from build123d import *

# Parameters (mm, degrees)
SKETCH1_W                    = 60
SKETCH1_H                    = 170
BASE_FLANGE1_DEPTH           = 4
EDGE_FLANGE1_STRIP_W         = 26
EDGE_FLANGE1_STRIP_H         = 4
EDGE_FLANGE1_STRIP_CUT_DEPTH = 170
EDGE_FLANGE1_DEPTH           = 170
SKETCH15_R                   = 15
SKETCH15_R_2                 = 10
CUT_EXTRUDE4_DEPTH           = 10
CUT_EXTRUDE5_DEPTH           = 10
SKETCH31_R                   = 2.6
CUT_EXTRUDE9_DEPTH           = 7
FILLET1_R                    = 10
SKETCH32_R                   = 1.6
CUT_EXTRUDE10_DEPTH          = 10
F_1_0MM_DOWEL_HOLE2_D        = 5.2
F_1_0MM_DOWEL_HOLE2_DEPTH    = 12.03
F_1_0MM_DOWEL_HOLE2_TIP      = 1.562237609
F_1_0MM_DOWEL_HOLE3_D        = 5.2
F_1_0MM_DOWEL_HOLE3_DEPTH    = 12.03
F_1_0MM_DOWEL_HOLE3_TIP      = 1.562237609
CUT_EXTRUDE11_DEPTH          = 10


# Sheet-metal steps are written as plain solids
with BuildPart() as part:
    # Sketch1 → Base-Flange1 (new body)
    with BuildSketch(Plane(origin=(0, 0, 0), x_dir=(1, 0, 0), z_dir=(0, 1, 0))):
        Rectangle(SKETCH1_W, SKETCH1_H)
    extrude(amount=-BASE_FLANGE1_DEPTH)

    # Edge-Flange1 strip (across the edge) → Edge-Flange1 strip cut (cut)
    with BuildSketch(Plane(origin=(30, 0, 85), x_dir=(-1, 0, 0), z_dir=(0, 0, -1))):
        with Locations((-8, -2)):
            Rectangle(EDGE_FLANGE1_STRIP_W, EDGE_FLANGE1_STRIP_H)
    extrude(amount=EDGE_FLANGE1_STRIP_CUT_DEPTH, mode=Mode.SUBTRACT)

    # Edge-Flange1 section (across the edge) → Edge-Flange1 (add)
    with BuildSketch(Plane(origin=(30, 0, 85), x_dir=(-1, 0, 0), z_dir=(0, 0, -1))):
        with BuildLine():
            Line((-4, 5), (-4, 186))
            Line((-4, 186), (0, 186))
            Line((0, 186), (0, 5))
            ThreePointArc((0, 5), (1.464466094, 1.464466094), (5, 0))
            Line((5, 0), (5, -4))
            ThreePointArc((5, -4), (-1.363961031, -1.363961031), (-4, 5))
        make_face()
    extrude(amount=EDGE_FLANGE1_DEPTH)

    # Sketch15 → Cut-Extrude4 (cut)
    with BuildSketch(Plane(origin=(34, 0, 0), x_dir=(0, 0, -1), z_dir=(1, 0, 0))):
        with Locations(Location((-43, 63, 0), (0, 0, 90))):
            Circle(SKETCH15_R)
        with Locations(Location((57, 143, 0), (0, 0, 90))):
            Circle(SKETCH15_R_2)
    extrude(amount=-CUT_EXTRUDE4_DEPTH, mode=Mode.SUBTRACT)

    # Sketch16 → Cut-Extrude5 (cut)
    with BuildSketch(Plane(origin=(34, 0, 0), x_dir=(0, 0, -1), z_dir=(1, 0, 0))):
        Polygon((-85, 186), (-85, 96), (45, 186), align=None)
    extrude(amount=-CUT_EXTRUDE5_DEPTH, mode=Mode.SUBTRACT)

    # Sketch31 → Cut-Extrude9 (cut)
    with BuildSketch(Plane.ZY.offset(-30)):
        with Locations(Location((76, 61.5, 0), (0, 0, 270))):
            Circle(SKETCH31_R)
        with Locations(Location((10, 61.5, 0), (0, 0, 270))):
            Circle(SKETCH31_R)
        with Locations(Location((43, 23, 0), (0, 0, 270))):
            Circle(SKETCH31_R)
    extrude(amount=-CUT_EXTRUDE9_DEPTH, mode=Mode.SUBTRACT)

    # Fillet1
    fillet1_edges = [part.edges().sort_by_distance(p)[0] for p in [
        (32, 186, -85),
        (32, 186, -45),
        (32, 96, 85),
        (-30, -2, 85),
        (-30, -2, -85),
    ]]
    fillet(fillet1_edges, radius=FILLET1_R)

    # Sketch32 → Cut-Extrude10 (cut)
    with BuildSketch(Plane.ZY.offset(-30)):
        with Locations(Location((-74.67766953, 143, 0), (0, 0, 270))):
            Circle(SKETCH32_R)
        with Locations(Location((-57, 125.32233047, 0), (0, 0, 270))):
            Circle(SKETCH32_R)
        with Locations(Location((-39.32233047, 143, 0), (0, 0, 270))):
            Circle(SKETCH32_R)
        with Locations(Location((-57, 160.67766953, 0), (0, 0, 270))):
            Circle(SKETCH32_R)
    extrude(amount=-CUT_EXTRUDE10_DEPTH, mode=Mode.SUBTRACT)

    # Ø1.0mm Dowel Hole2
    with Locations(Plane(origin=(34, 0, 0), x_dir=(0, 0, -1), z_dir=(1, 0, 0))):
        with Locations((-72.5, 26), (72.5, 26), (72.5, 116), (-22.5, 101), (59.5, 178)):
            Hole(F_1_0MM_DOWEL_HOLE2_D / 2, depth=F_1_0MM_DOWEL_HOLE2_DEPTH)
            with Locations((0, 0, -(F_1_0MM_DOWEL_HOLE2_DEPTH + F_1_0MM_DOWEL_HOLE2_TIP / 2))):  # 118° drill point
                Cone(0, F_1_0MM_DOWEL_HOLE2_D / 2, F_1_0MM_DOWEL_HOLE2_TIP, mode=Mode.SUBTRACT)

    # Ø1.0mm Dowel Hole3
    with Locations(Plane(origin=(0, 0, 0), x_dir=(1, 0, 0), z_dir=(0, 1, 0))):
        with Locations((-15, 70), (-15, 0), (-15, -70)):
            Hole(F_1_0MM_DOWEL_HOLE3_D / 2, depth=F_1_0MM_DOWEL_HOLE3_DEPTH)
            with Locations((0, 0, -(F_1_0MM_DOWEL_HOLE3_DEPTH + F_1_0MM_DOWEL_HOLE3_TIP / 2))):  # 118° drill point
                Cone(0, F_1_0MM_DOWEL_HOLE3_D / 2, F_1_0MM_DOWEL_HOLE3_TIP, mode=Mode.SUBTRACT)

    # Sketch40 → Cut-Extrude11 (cut)
    with BuildSketch(Plane(origin=(0, 0, 0), x_dir=(1, 0, 0), z_dir=(0, 1, 0))):
        with BuildLine():
            Line((-19, -72.6), (-11, -72.6))
            ThreePointArc((-11, -72.6), (-8.4, -70), (-11, -67.4))
            Line((-11, -67.4), (-19, -67.4))
            ThreePointArc((-19, -67.4), (-21.6, -70), (-19, -72.6))
        make_face()
        with BuildLine():
            Line((-19, -2.6), (-11, -2.6))
            ThreePointArc((-11, -2.6), (-8.4, 0), (-11, 2.6))
            Line((-11, 2.6), (-19, 2.6))
            ThreePointArc((-19, 2.6), (-21.6, 0), (-19, -2.6))
        make_face()
        with BuildLine():
            Line((-19, 67.4), (-11, 67.4))
            ThreePointArc((-11, 67.4), (-8.4, 70), (-11, 72.6))
            Line((-11, 72.6), (-19, 72.6))
            ThreePointArc((-19, 72.6), (-21.6, 70), (-19, 67.4))
        make_face()
    extrude(amount=-CUT_EXTRUDE11_DEPTH, mode=Mode.SUBTRACT)


solid = part.part
Can you work these out from the model? Positions are in its coordinate system, mm. A direction names the side the tool comes from. Round coordinates to 2 decimals unless told otherwise and drop trailing zeros. Loops run counter-clockwise (first coordinate to the right, second up) from the corner with the lowest first, then second, coordinate; pieces in that order, holes last. Notation, with made-up numbers: (4.5, 49) - (42.5, 49) arc R32 ccw to (42.5, 76) - close; hole circle Ø5 at (-13.75, 57.5). An arc over 180 degrees is marked (long way). Answer in a Markdown table with one row per item. Add a question column.
Q1. We'd pull the mould along Z, two halves only. Please class faces 4 (the cylindrical face through (-8.4, -2, 70.1)), 5 (the cylindrical face through (-26.99, -2.03, -82.15)), 6 (the flat face through (30, 77, -18)): pulls with the +Z half, pulls with the -Z half, needs draft (parallel to the pull), parting line crosses it, or undercut.
Q2. I want a section at C-C on z = 30.5. List the corners of the cut face in (x, y) for me, and give its area (3 significant figures).
Q3. I need wall thicknesses on L1, parallel to Z at x = 32.25, y = 23; L2, parallel to Z at x = 31.7, y = 61.5; L3, parallel to Y at x = 32.35, z = -59.5. Which ranges of each line are inside material? Lowest first, please.
Q4. Which directions (+Z, -Z, +X, -X, +Y, -Y) give clear straight access to the entire face, cutting with the end or side of a thin tool? Please do faces 1 (the flat face through (-3, 0, -1)), 2 (the flat face through (-3, -4, -1)), 3 (the cylindrical face through (-8.4, -2, -69.9)).
Q5. For pin 1 Ø5 at (y, z) = (160.68, -57) entering from -X; pin 2 Ø16.5 at (x, z) = (9.5, -35) entering from +Y; pin 3 Ø3.5 at (y, z) = (143, -74.68) entering from +X, each with a flat end and sliding along its axis, tell me the tip position at first contact or that it passes through.
Q6. I want a section at B-B on y = 147. List the corners of the cut face in (x, z) for me.
Q7. I want a section at D-D on y = 70.5. List the corners of the cut face in (x, z) for me, and give its area (3 significant figures).
Q8. I want a section at A-A on z = -25.5. List the corners of the cut face in (x, y) for me, and give its area (3 significant figures).
A:
| question | item | result |
|---|---|---|
| 1 | face 4 | undercut |
| 1 | face 5 | pulls with the -Z half |
| 1 | face 6 | needs draft |
| 2 | outline | (-30, -4) - (25, -4) arc R9 ccw to (34, 5) - (34, 54.71) - (30, 54.71) - (30, 5) arc R5 cw to (25, 0) - (-30, 0) - close; (30, 71.29) - (34, 71.29) - (34, 133.73) - (30, 133.73) - close |
| 2 | area | 713 mm^2 |
| 3 | L1 | -85 to 40.4, 45.6 to 85 |
| 3 | L2 | -85 to 7.4, 12.6 to 28.08, 57.92 to 73.4, 78.6 to 85 |
| 3 | L3 | -0.19 to 133.32, 152.68 to 175.4, 180.6 to 186 |
| 4 | face 1 | +Z, -Z, -X, +Y |
| 4 | face 2 | +Z, -Z, +X, -X, -Y |
| 4 | face 3 | +Y, -Y |
| 5 | pin 1 | x = 30 |
| 5 | pin 2 | y = 0 |
| 5 | pin 3 | x = 34 |
| 6 | outline | (30, -85) - (34, -85) - (34, -66.17) - (30, -66.17) - close; (30, -47.83) - (34, -47.83) - (34, 11.33) - (30, 11.33) - close |
| 7 | outline | (30, -85) - (34, -85) - (34, 30.01) - (30, 30.01) - close; (30, 55.99) - (34, 55.99) - (34, 85) - (30, 85) - close |
| 7 | area | 576 mm^2 |
| 8 | outline | (-30, -4) - (25, -4) arc R9 ccw to (34, 5) - (34, 172.5) - (30, 172.5) - (30, 5) arc R5 cw to (25, 0) - (-30, 0) - close |
| 8 | area | 934 mm^2 |
